```python
from build123d import *

# Parameters (mm, degrees)
PROFILEBOSS_EXTRUDE1_DEPTH      = 110
SKETCH3_R                       = 2.3
MOUNTINGHOLESCUT_EXTRUDE3_DEPTH = 4.5
XAXISCABLECUT_EXTRUDE1_DEPTH    = 4.25


with BuildPart() as part:
    # Sketch1 → ProfileBoss-Extrude1 (new body)
    with BuildSketch(Plane(origin=(0, 0, 0), x_dir=(0, 0, -1), z_dir=(1, 0, 0))):
        with BuildLine():
            Line((0, 0), (5.499461553, 0))
            ThreePointArc((5.499461553, 0), (6.914055855, 0.585944145), (7.5, 2.000538447))
            Line((7.5, 2.000538447), (7.5, 3.5))
            Line((7.5, 3.5), (17.922539551, 8.36011001))
            Line((17.922539551, 8.36011001), (19.190394336, 5.641186649))
            ThreePointArc((19.190394336, 5.641186649), (20.700753359, 6.16912635), (21.340729536, 7.635528477))
            Line((21.340729536, 7.635528477), (21.340729536, 13.36011001))
            ThreePointArc((21.340729536, 13.36011001), (20.754943098, 14.774323572), (19.340729536, 15.36011001))
            Line((19.340729536, 15.36011001), (0, 15.36011001))
            Line((0, 15.36011001), (0, 0))
        make_face()
    extrude(amount=PROFILEBOSS_EXTRUDE1_DEPTH)

    # Sketch3 → MountingHolesCut-Extrude3 (cut)
    with BuildSketch(Plane.XY):
        with Locations((55, 10.86011001)):
            Circle(SKETCH3_R)
    extrude(amount=-MOUNTINGHOLESCUT_EXTRUDE3_DEPTH, mode=Mode.SUBTRACT)

    # Sketch4 → XAxisCableCut-Extrude1 (cut)
    with BuildSketch(Plane.XY):
        with BuildLine():
            Line((55, 4.5), (110, 4.5))
            Line((110, 4.5), (110, 2.5))
            Line((110, 2.5), (56.872897785, 2.5))
            ThreePointArc((56.872897785, 2.5), (55.642642805, 1.25), (56.872897785, 0))
            Line((56.872897785, 0), (48.989527283, 0))
            ThreePointArc((48.989527283, 0), (51.20727122, 0.684547643), (52.653343966, 2.5))
            ThreePointArc((52.653343966, 2.5), (53.458345487, 3.932167796), (55, 4.5))
        make_face()
    extrude(amount=-XAXISCABLECUT_EXTRUDE1_DEPTH, mode=Mode.SUBTRACT)


solid = part.part
```
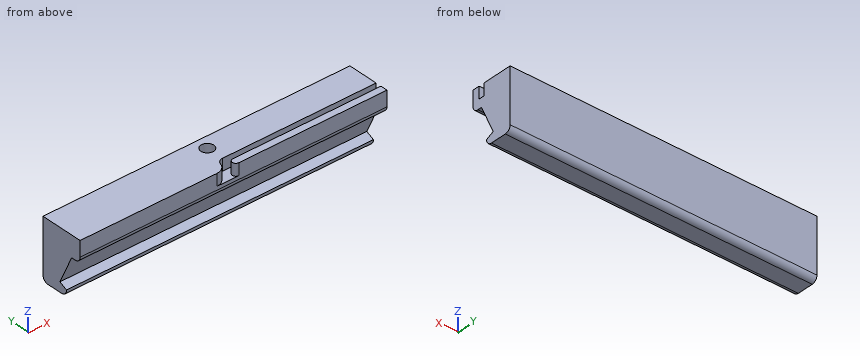
Here's how the part is built. I have some questions about the finished solid (model axes, mm). Coordinates: 2 decimals unless noted, no trailing zeros. Loops run counter-clockwise (first coordinate to the right, second up) from the corner with the lowest first, then second, coordinate; pieces in that order, holes last. Notation, with made-up numbers: M 30.5,20.25 L 61.5,20.25 A14 ccw 61.5,25.25 Z; hole C 57,-16 d11. An arc over 180 degrees is marked long. One line per item, written item: value.
1. Imagine slicing it at A-A (x = 90.5). List the corners of the cut face in (y, z) for me.
Geometry says:
outline: M 0,-5.5 A2 ccw 2,-7.5 L 3.5,-7.5 L 8.36,-17.92 L 5.64,-19.19 A2 ccw 7.64,-21.34 L 13.36,-21.34 A2 ccw 15.36,-19.34 L 15.36,0 L 4.5,0 L 4.5,-4.25 L 2.5,-4.25 L 2.5,0 L 0,0 Z
2. Will these pins go through, and if not, where does the flat tip stop? pin 1 Ø1.6 at (x, y) = (73, 3) entering from -Z; pin 2 Ø3.5 at (x, y) = (55, 10.86) entering from +Z.
Geometry says:
pin 1: stops at z = -8.14
pin 2: stops at z = -4.5
3. Please list where these lines run through material, in increasing order: probe 1 along Y at (x, z) = (55, -1.4); probe 2 along Y at (x, z) = (63, -3.5); probe 3 along Z at (x, y) = (82, 2).
Geometry says:
probe 1: y = 4.5 to 8.56, 13.16 to 15.36
probe 2: y = 0 to 2.5, 4.5 to 15.36
probe 3: z = -7.5 to 0
4. Imagine slicing it at C-C (z = -9). List the corners of the cut face in (x, y) for me, and give its area (3 significant figures).
Geometry says:
outline: M 0,4.2 L 110,4.2 L 110,15.36 L 0,15.36 Z
area: 1,230 mm2
5. Imagine slicing it at B-B (x = 22). List the corners of the cut face in (y, z) for me, and give its area (3 significant figures).
Geometry says:
outline: M 0,-5.5 A2 ccw 2,-7.5 L 3.5,-7.5 L 8.36,-17.92 L 5.64,-19.19 A2 ccw 7.64,-21.34 L 13.36,-21.34 A2 ccw 15.36,-19.34 L 15.36,0 L 0,0 Z
area: 242 mm2
